Solid Edge part; units mm, degrees
sketch "Sketch1" plane through (0, 0, 0) normal (0, -1, 0) x (1, 0, 0)
  circle A0 centre (0, 0) radius 1.5
extrude "Protrusion1" add sketch "Sketch1" along normal mid plane 30
sketch "Sketch2" plane through (0, 15, 0) normal (0, 1, 0) x (1, 0, 0)
  line L0 (0, 1.5) -> (-2, 1.5)
  line L1 (-2, 1.5) -> (-2, -1.5)
  line L2 (-2, -1.5) -> (2, -1.5)
  line L3 (2, -1.5) -> (2, 1.5)
  line L4 (2, 1.5) -> (0, 1.5)
extrude "ExtrudedProtrusion_2" add sketch "Sketch2" against normal blind 4
hole "Hole_1" at (0, 13, 1.5) direction (0, 0, -1) diameter 2.1565 end up to next thread major 2.8448 thread length 50.8
fillet "Round_1" radius 2 2 edges at (-2, 15, 0) (2, 15, 0)
properties material "Aluminum, 6061-T6"
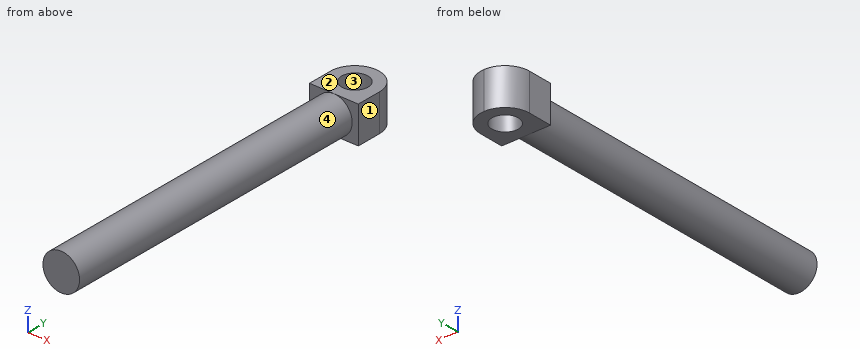
Read the model definition and answer for the solid it produces. Units are mm, in the model's axes. Face numbers are marked on the shaded views. Coordinates: 2 decimals unless noted, no trailing zeros. Order: outer loops, then holes, each group sorted by start corner. A loop starts at its lowest first (then second) coordinate and runs counter-clockwise, first axis right, second up. Notation, with made-up numbers: (60, -14) -> (109, -14) arc R35 ccw to (109, 19) -> close; hole circle Ø9 at (8.25, 46). An arc over 180 degrees is marked (long way). Answer as a JSON object with one key per item and string values.
1) Consider line 1 along Y through (x, z) = (0, -0.5); line 2 along X through (y, z) = (13, 0.55); line 3 along Y through (x, z) = (-0.6, -0.75). Determine where each line is inside the solid, lowest interval first. Write a range as from..to.
Model answer:
{"line 1": "y = -15..11.92, 14.08..15", "line 2": "x = -2..-1.08, 1.08..2", "line 3": "y = -15..12.1, 13.9..14.91"}
2) Each of these flat-tipped pins is pushed along its axis until it touches: pin 1 (1.5 mm diameter, centred on y = -1, z = -1, fed in from -X); pin 2 (1 mm diameter, centred on y = -11, z = 1, fed in from +X). Where does it stop, or does it pass through?
Model answer:
{"pin 1": "stops at x = -1.48", "pin 2": "stops at x = 1.41"}
3) The mould has two halves that part along X. Classify the marked faces 1, 2, 3 and 4: released by +X, released by -X, zero draft, split by the parting line, or undercut.
Model answer:
{"face 1": "released by +X", "face 2": "zero draft", "face 3": "undercut", "face 4": "split by the parting line"}
4) A cutting plane is placed at C-C, the plane y = 9.25. Determine the outline of the cut face in (x, z).
Model answer:
{"outline": "circle Ø3 at (0, 0)"}
